Input: part model. Units: mm. Frame: model coordinates. A direction names the side the tool comes from. Coordinates: 2 decimals unless noted, no trailing zeros. Loops run counter-clockwise (first coordinate to the right, second up) from the corner with the lowest first, then second, coordinate; pieces in that order, holes last.
(1) Section D-D, the plane x = -9.5. Return loops of the section in (y, z).
(2) Mould query, pull axis X, two halves, no side actions, for faces 4 (the face through (15.466, 13.832, 2.218)), 5 (the face through (23.846, 7.509, 2.218)), 6 (the face through (-9.769, -0.751, 14.885)). Classes: released by +X, released by -X, zero draft, split by the parting line, or undercut.
(3) Section A-A, the plane x = 0. Return loops of the section in (y, z), then the cut area to 3 significant figures.
(4) Line query: L1, parallel to Y at x = 0, z = 1; L2, parallel to Z at x = -14, y = -3; L3, parallel to Y at x = 4.5, z = 16.5. Output: solid intervals per line, ascending.
(5) Section C-C, the plane z = 12.5. Return loops of the section in (x, y).
(6) Set-up query: faces 1 (the face through (0.751, -9.763, 14.885)), 2 (the face through (-6, -11, 4.5)), 3 (the face through (-13.4, -10.6, 2.2)). Return all of +Z, -Z, +X, -X, +Y, -Y with unobstructed straight access to the full face (end or side cutting, diameter ignored); none if empty.
(7) Contact query for flat-ended pins moving along their axis: P1, Ø6.5, axis at x = 13.08, y = -13.08, coming from the +Z side; P2, Ø3, axis at y = -15.5, z = 4, coming from the +X side; P3, Ø6, axis at y = 0, z = 12.5, coming from the +X side. Output: stop coordinate, or through.
```python
from build123d import *

# Parameters (mm, degrees)
SKETCH_1_R          = 25
SKETCH_1_R_2        = 8
SKETCH_1_R_3        = 2.5
EXTRUDE_1_DEPTH     = 4.5
SKETCH_2_R          = 12
SKETCH_2_R_2        = 8
EXTRUDE_2_DEPTH     = 13
SKETCH_3_R          = 2.5
CUT_EXTRUDE_1_DEPTH = 26
SKETCH_5_R          = 2.5
CUT_EXTRUDE_4_DEPTH = 26


with BuildPart() as part:
    # 草图1 → 凸台-拉伸1 (new body)
    with BuildSketch(Plane.XY):
        Circle(SKETCH_1_R)
        Circle(SKETCH_1_R_2, mode=Mode.SUBTRACT)
        with Locations((13.081475452, 13.081475452)):
            Circle(SKETCH_1_R_3, mode=Mode.SUBTRACT)
        with Locations((13.081475452, -13.081475452)):
            Circle(SKETCH_1_R_3, mode=Mode.SUBTRACT)
        with Locations((-13.081475452, -13.081475452)):
            Circle(SKETCH_1_R_3, mode=Mode.SUBTRACT)
        with Locations((-13.081475452, 13.081475452)):
            Circle(SKETCH_1_R_3, mode=Mode.SUBTRACT)
    extrude(amount=EXTRUDE_1_DEPTH)

    # 草图2 → 凸台-拉伸2 (add)
    with BuildSketch(Plane.XY.offset(4.5)):
        with Locations(Location((0, 0, 0), (0, 0, 180))):
            Circle(SKETCH_2_R)
        Circle(SKETCH_2_R_2, mode=Mode.SUBTRACT)
    extrude(amount=EXTRUDE_2_DEPTH)

    # 草图3 → 切除-拉伸1 (cut)
    with BuildSketch(Plane(origin=(0, 0, 0), x_dir=(1, 0, 0), z_dir=(0, 1, 0))):
        with Locations(Location((0, -12.5, 0), (0, 0, 270))):
            Circle(SKETCH_3_R)
    extrude(amount=-CUT_EXTRUDE_1_DEPTH, mode=Mode.SUBTRACT)

    # 草图5 → 切除-拉伸4 (cut)
    with BuildSketch(Plane(origin=(0, 0, 0), x_dir=(0, 0, -1), z_dir=(1, 0, 0))):
        with Locations(Location((-12.5, 0, 0), (0, 0, 180))):
            Circle(SKETCH_5_R)
    extrude(amount=-CUT_EXTRUDE_4_DEPTH, mode=Mode.SUBTRACT)


solid = part.part
```
Report:
1. outline: (-23.12, 0) - (23.12, 0) - (23.12, 4.5) - (7.33, 4.5) - (7.33, 17.5) - (-7.33, 17.5) - (-7.33, 4.5) - (-23.12, 4.5) - close; hole circle Ø5 at (0, 12.5)
2. face 4: undercut
2. face 5: split by the parting line
2. face 6: zero draft
3. outline: (-25, 0) - (-8, 0) - (-8, 10) - (-12, 10) - (-12, 4.5) - (-25, 4.5) - close; (-12, 15) - (-8, 15) - (-8, 17.5) - (-12, 17.5) - close; (8, 0) - (25, 0) - (25, 4.5) - (12, 4.5) - (12, 17.5) - (8, 17.5) - close
3. area: 237 mm2
4. L1: y = -25 to -8, 8 to 25
4. L2: z = 0 to 4.5
4. L3: y = -11.12 to -6.61, 6.61 to 11.12
5. outline: (-11.74, -2.5) arc R12 ccw to (-2.5, -11.74) - (-2.5, -7.6) arc R8 cw to (-7.6, -2.5) - close; (-11.74, 2.5) - (-7.6, 2.5) arc R8 cw (long way) to (2.5, -7.6) - (2.5, -11.74) arc R12 ccw (long way) to start
6. face 1: -Y
6. face 2: +Z
6. face 3: +Z, -Z
7. P1: stops at z = 4.5
7. P2: stops at x = 20.71
7. P3: stops at x = 12
